Study the drawing (mm; zero at the part's minimum x, y, z) and answer. Coordinates: 2 decimals unless noted, no trailing zeros. Loops run counter-clockwise (first coordinate to the right, second up) from the corner with the lowest first, then second, coordinate; pieces in that order, holes last.
Q1. Section B-B (z = 4.5) is taken. Give the vertices of the cut face in (x, y).
Q2. Flat-ended cylindrical pins translate along their axes: P1, Ø0.6, axis at x = 13.5, y = 1.5, coming from the +Z side; P2, Ø0.6, axis at y = 1, z = 28, coming from the +X side; P3, Ø1, axis at y = 1, z = 2, coming from the +X side. Find the tip coordinate at first contact, or state that the pin passes through.
Q3. Section A-A (y = 1.7) is taken. Give the vertices of the cut face in (x, z), then the cut area to 4 significant figures.
Q4. Straight lines are drawn through the part: line 1 (Z direction, x = 18.25, y = 0.2); line 2 (X direction, y = 1.4, z = 27.75); line 3 (Z direction, x = 6.25, y = 0.65). For each, find the intervals that lie inside material, in ascending order.
Q5. Section C-C (x = 10.25) is taken. Give the vertices of the cut face in (y, z), then the cut area to 3 significant figures.
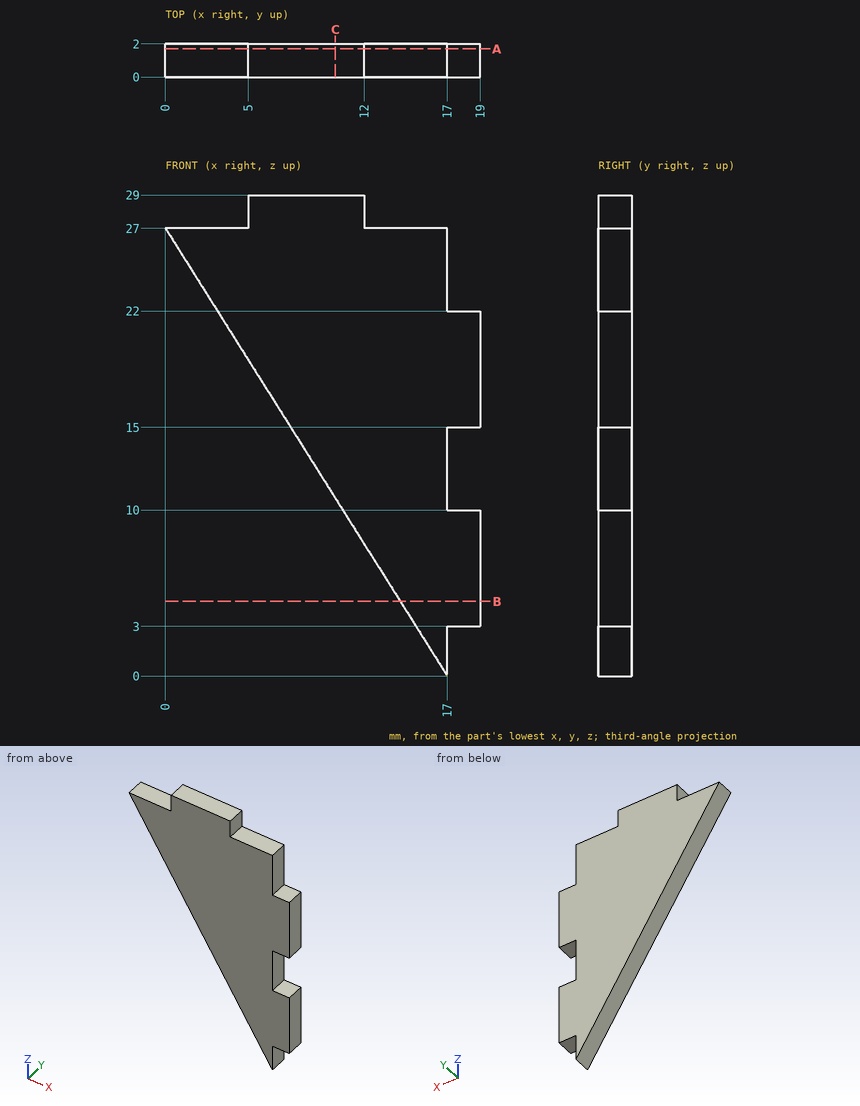
Numbers:
1. outline: (14.17, 0) - (19, 0) - (19, 2) - (14.17, 2) - close
2. P1: stops at z = 27
2. P2: stops at x = 12
2. P3: stops at x = 17
3. outline: (0, 27) - (17, 0) - (17, 3) - (19, 3) - (19, 10) - (17, 10) - (17, 15) - (19, 15) - (19, 22) - (17, 22) - (17, 27) - (12, 27) - (12, 29) - (5, 29) - (5, 27) - close
3. area: 271.5 mm2
4. line 1: z = 3 to 10, 15 to 22
4. line 2: x = 5 to 12
4. line 3: z = 17.07 to 29
5. outline: (0, 10.72) - (2, 10.72) - (2, 29) - (0, 29) - close
5. area: 36.6 mm2
